Autodesk Fusion 360 part; units mm, degrees
sketch "Sketch1" plane through (0, 0, 0) normal (0, 0, 1) x (1, 0, 0) in component "Cover"
  line L0 (20, 20) -> (128, 20)
  line L1 (128, 20) -> (128, 135)
  line L2 (128, 135) -> (20, 135)
  line L3 (20, 135) -> (20, 20)
  dimension "d1" = 20
  dimension "d2" = 20
  dimension "d3" = 115
  dimension "d4" = 108
extrude "Extrude1" add sketch "Sketch1" along normal blind 20 in component "Cover"
sketch "Sketch2" plane through (0, 0, 0) normal (0, 0, -1) x (-1, 0, 0) in component "Cover"
  line L0 (-20, 20) -> (-20, 135)
  line L1 (-20, 135) -> (-128, 135)
  line L2 (-128, 135) -> (-128, 20)
  line L3 (-128, 20) -> (-20, 20)
  line L4 (-126, 104) -> (-22, 104)
  line L5 (-22, 104) -> (-22, 22)
  line L6 (-22, 22) -> (-126, 22)
  line L7 (-126, 22) -> (-126, 104)
  dimension "d8" = 2
  dimension "d10" = 2
  dimension "d28" = 82
  dimension "d29" = 104
extrude "Extrude2" cut sketch "Sketch2" against normal blind 18 contours L4 L5 L6 L7 in component "Cover"
sketch "Sketch3" plane through (20, 0, 0) normal (-1, 0, 0) x (0, 0, 1) in component "Cover"
  line L0 (0, 135) -> (0, 20)
  line L1 (0, 20) -> (20, 20)
  line L2 (20, 20) -> (20, 135)
  line L3 (20, 135) -> (0, 135)
  line L4 (0, 58) -> (14, 58)
  line L5 (14, 58) -> (14, 42)
  line L6 (14, 42) -> (0, 42)
  line L7 (20, 135) -> (0, 135)
  line L8 (0, 135) -> (20, 127)
  line L9 (0, 120) -> (3, 120)
  line L10 (3, 120) -> (3, 110)
  line L11 (3, 110) -> (0, 110)
  line L12 (0, 110) -> (0, 120)
  line L13 (0, 70) -> (3, 70)
  line L14 (3, 70) -> (3, 60)
  line L15 (3, 60) -> (0, 60)
  line L16 (0, 60) -> (0, 70)
  dimension "d13" = 14
  dimension "d14" = 16
  dimension "d16" = 22
  dimension "d30" = 8
  dimension "d51" = 3
  dimension "d52" = 10
  dimension "d53" = 3
  dimension "d54" = 10
  dimension "d55" = 90
  dimension "d56" = 40
sketch "Sketch1 (2)" plane through (0, 20, 0) normal (0, -1, 0) x (1, 0, 0)
  line L0 (20, 0) -> (128, 0)
  line L1 (128, 0) -> (128, 20)
  line L2 (128, 20) -> (20, 20)
  line L3 (20, 20) -> (20, 0)
  line L4 (95, 5) -> (107, 5)
  line L5 (107, 5) -> (107, 10)
  line L6 (107, 10) -> (95, 10)
  line L7 (95, 10) -> (95, 5)
  point P0 (20, 0)
  dimension "d22" = 5
  dimension "d23" = 12
  dimension "d24" = 75
  dimension "d25" = 5
extrude "Extrude6" cut sketch "Sketch3" against normal up to surface (108 mm away) contours L2 L3 L7 L8 in component "Cover"
sketch "Sketch2 (2)" plane through (0, 0, 0) normal (0, 0, -1) x (-1, 0, 0)
  line L0 (-22, 104) -> (-22, 22)
  line L1 (-22, 22) -> (-126, 22)
  line L2 (-126, 22) -> (-126, 104)
  line L3 (-126, 104) -> (-22, 104)
  line L4 (-20, 20) -> (-20, 135)
  line L5 (-20, 135) -> (-128, 135)
  line L6 (-128, 135) -> (-128, 20)
  line L7 (-128, 20) -> (-20, 20)
  line L8 (-104, 104) -> (-80, 104)
  line L9 (-80, 104) -> (-80, 125)
  line L10 (-80, 125) -> (-104, 125)
  line L11 (-104, 125) -> (-104, 104)
  line L12 (-104, 125) -> (-80, 125)
  line L13 (-80, 125) -> (-80, 135)
  line L14 (-80, 135) -> (-104, 135)
  line L15 (-104, 135) -> (-104, 125)
  dimension "d33" = 21
  dimension "d34" = 24
  dimension "d35" = 22
  dimension "d36" = 24
extrude "Extrude7" cut sketch "Sketch2 (2)" against normal up to surface (18 mm away) contours L3 L8 L9 L10 L11 L12 in component "Cover"
extrude "Extrude8" cut sketch "Sketch2 (2)" against normal blind 2 contours L5 L10 L12 L13 L14 L15 in component "Cover"
extrude "Extrude9" cut sketch "Sketch3" against normal up to surface (2 mm away) contours L0 L4 L5 L6 in component "Cover"
sketch "Sketch3 (2)" plane through (128, 0, 0) normal (1, 0, 0) x (0, 0, -1)
  line L0 (0, 135) -> (-20, 127)
  line L1 (-20, 127) -> (-20, 20)
  line L2 (-20, 20) -> (0, 20)
  line L3 (0, 20) -> (0, 135)
  line L4 (0, 120) -> (-3, 120)
  line L5 (-3, 120) -> (-3, 110)
  line L6 (-3, 110) -> (0, 110)
  line L7 (0, 110) -> (0, 120)
  line L8 (0, 60) -> (-3, 60)
  line L9 (-3, 60) -> (-3, 50)
  line L10 (-3, 50) -> (0, 50)
  line L11 (0, 50) -> (0, 60)
  dimension "d43" = 3
  dimension "d44" = 10
  dimension "d45" = 10
  dimension "d46" = 3
  dimension "d47" = 30
  dimension "d48" = 50
extrude "Extrude10" add sketch "Sketch3 (2)" along normal blind 10 contours L3 L4 L5 L6 L7 | L3 L8 L9 L10 L11 in component "Cover"
extrude "Extrude11" add sketch "Sketch3" along normal blind 10 contours L0 L9 L10 L11 L12 | L0 L13 L14 L15 L16 in component "Cover"
component "Cover" placed x (1, 0, 0) y (0, 1, 0) z (0, 0, 1) at (0, 0, 0)
Source: CAD feature listing. Evaluate the final solid. Frame: model axes, mm. A direction names the side the tool comes from. Round coordinates to 2 decimals unless told otherwise and drop trailing zeros. Write each loop counter-clockwise with the first axis right and the second up, starting at its lowest first coordinate (ties: lowest second). Pieces come first, ordered by that corner, then holes. Notation, with made-up numbers: M 17.25,-36.5 L 38.25,-36.5 A22 ccw 38.25,-0.5 Z; hole C -1,45.5 d9. An arc over 180 degrees is marked long. One line per item, written item: value. Start each with the question number.
Item 1: Section query C-C (z = 7.75). Return the cut outline in (x, y).
Item 2: Pin query (flat end, axial travel): pin 1 (11 mm diameter, centred on x = 135, y = 55, fed in from +Z); pin 2 (2 mm diameter, centred on x = 80.5, y = 88.5, fed in from -Z); pin 3 (4 mm diameter, centred on y = 93.5, z = 14, fed in from -X). Return the tip coordinate at first contact, or that it passes through.
Item 3: Section query D-D (y = 48). Return the cut outline in (x, z), plus the area to 3 significant figures.
Item 4: Section query B-B (z = 16.25). Return the cut outline in (x, y), plus the area to 3 significant figures.
Item 5: Set-up query: faces 4 (the flat face through (15, 70, 1)), 5 (the flat face through (104, 116, 9)), 6 (the flat face through (15, 60, 2)), 7 (the flat face through (133, 115, 3)), 8 (the flat face through (15, 120, 1)). Return all of +Z, -Z, +X, -X, +Y, -Y with unobstructed straight access to the full face (end or side cutting, diameter ignored); none if empty.
Item 6: Section query A-A (x = 130). Return the cut outline in (y, z).
Item 7: Mould query, pull axis X, two halves, no side actions, for faces 1 (the flat face through (73, 74, 20)), 2 (the flat face through (73, 22, 9)), 3 (the flat face through (138, 55, 2)). Classes: pulls with the +X half, pulls with the -X half, needs draft (parallel to the pull), parting line crosses it, or undercut.
Item 8: Ray query, L1, parallel to X at y = 74.5, z = 11.75; L2, parallel to X at y = 110, z = 13.5; L3, parallel to Z at x = 95.5, y = 59.5. Return the intervals inside material, ascending. Write a range as from..to.
Result set:
1. outline: M 20,20 L 128,20 L 128,131.9 L 20,131.9 L 20,58 L 22,58 L 22,104 L 80,104 L 80,125 L 104,125 L 104,104 L 126,104 L 126,22 L 22,22 L 22,42 L 20,42 Z
2. pin 1: stops at z = 3
2. pin 2: stops at z = 18
2. pin 3: stops at x = 20
3. outline: M 20,14 L 22,14 L 22,18 L 126,18 L 126,0 L 128,0 L 128,20 L 20,20 Z
3. area: 260 mm²
4. outline: M 20,20 L 128,20 L 128,128.5 L 20,128.5 Z; hole M 22,22 L 126,22 L 126,104 L 104,104 L 104,125 L 80,125 L 80,104 L 22,104 Z
4. area: 2,690 mm²
5. face 4: +Z, -Z, -X
5. face 5: -Z
5. face 6: +Z, -Z, -X, -Y
5. face 7: +Z, +X, +Y, -Y
5. face 8: +Z, -Z, -X, +Y
6. outline: M 50,0 L 60,0 L 60,3 L 50,3 Z; M 110,0 L 120,0 L 120,3 L 110,3 Z
7. face 1: needs draft
7. face 2: undercut
7. face 3: pulls with the +X half
8. L1: x = 20..22, 126..128
8. L2: x = 20..80, 104..128
8. L3: z = 18..20
